Geometry check sheet. Reference: drawing and pictorial views, mm from the part's lowest x, y, z. A direction names the side the tool comes from. Give positions to 0.01 mm unless a question says otherwise; leave off trailing zeros. Order: outer loops, then holes, each group sorted by start corner. A loop starts at its lowest first (then second) coordinate and runs counter-clockwise, first axis right, second up. Notation, with made-up numbers: (67.5, -38.5) -> (97.5, -38.5) arc R33 ccw to (97.5, -0.5) -> close; hole circle Ø4 at (43, -36). An arc over 180 degrees is marked (long way). Write each question's results on one line, items separated by ' | '.
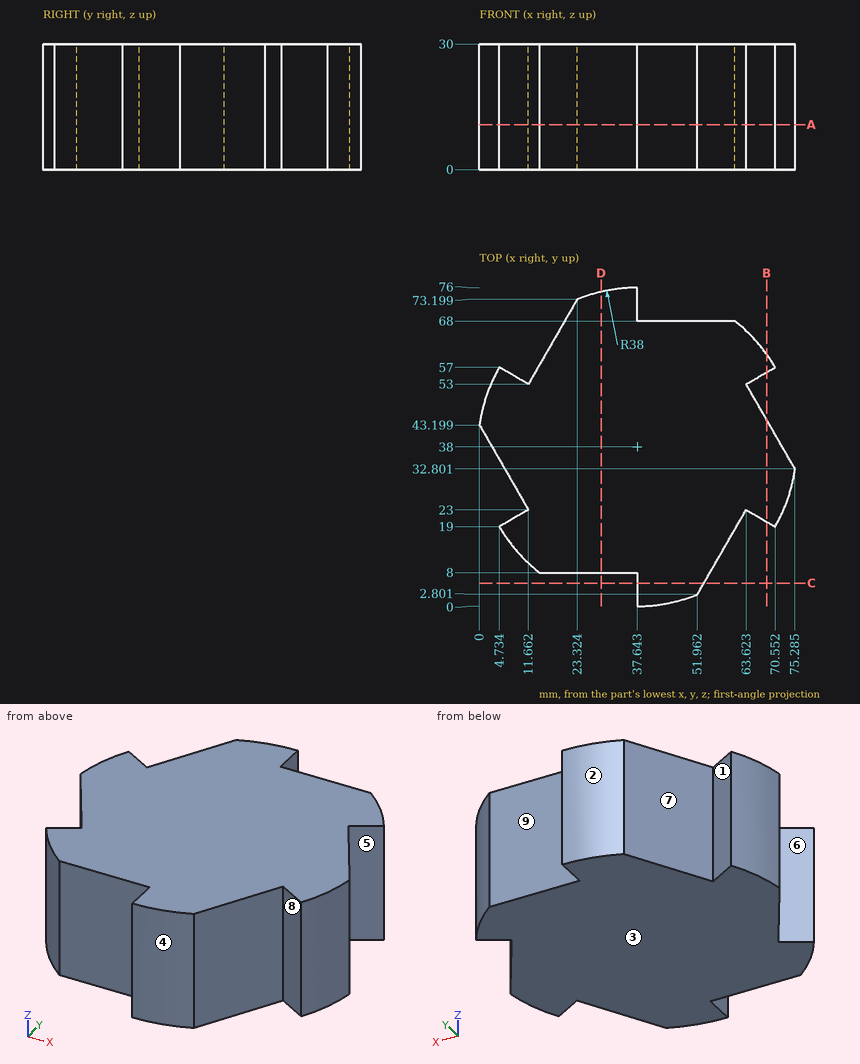
1. Mould release check, pull along X, two halves, no side actions. Record for the marked faces 1, 2, 3 and 4: +X half, -X half, draft (parallel to the pull), parting line (faces both ways), or undercut.
Verdict:
face 1: undercut | face 2: -X half | face 3: draft | face 4: +X half
2. Section check A-A on z = 10.75. Record the cut outline in (x, y) (1 decimal).
Verdict:
outline: (0, 43.2) -> (11.7, 23) -> (4.7, 19) arc R38 ccw to (14.3, 8) -> (37.6, 8) -> (37.6, 0) arc R38 ccw to (52, 2.8) -> (63.6, 23) -> (70.6, 19) arc R38 ccw to (75.3, 32.8) -> (63.6, 53) -> (70.6, 57) arc R38 ccw to (61, 68) -> (37.6, 68) -> (37.6, 76) arc R38 ccw to (23.3, 73.2) -> (11.7, 53) -> (4.7, 57) arc R38 ccw to start
3. Section check C-C on y = 5.5. Record the cut outline in (x, z).
Verdict:
outline: (37.64, 0) -> (53.52, 0) -> (53.52, 30) -> (37.64, 30) -> close
4. Gauge pin test, flat ends, axial feed: pin 1 Ø4 at (y, z) = (53.5, 16.5) entering from +X (1 decimal); pin 2 Ø2.5 at (y, z) = (72, 9) entering from +X; pin 3 Ø8 at (x, z) = (57.5, 7.5) entering from +Y. Record the tip position at first contact, or that the pin passes through.
Verdict:
pin 1: stops at x = 68 | pin 2: stops at x = 37.64 | pin 3: stops at y = 68
5. Material ranges on probe 1 along X at (y, z) = (21, 14.5) (1 decimal); probe 2 along Y at (x, z) = (70, 26.5) (1 decimal); probe 3 along Y at (x, z) = (8, 19) (1 decimal), recorded low to high. Write a range as from..to.
Verdict:
probe 1: x = 8.2..62.5, 67.1..71.6 | probe 2: y = 19.3..42, 56.7..57.9 | probe 3: y = 14.2..20.9, 29.3..55.1
6. Section check B-B on x = 68.5. Record the cut outline in (y, z) (1 decimal).
Verdict:
outline: (20.2, 0) -> (44.6, 0) -> (44.6, 30) -> (20.2, 30) -> close; (55.8, 0) -> (60.2, 0) -> (60.2, 30) -> (55.8, 30) -> close
7. Section check D-D on x = 29. Record the cut outline in (y, z) (1 decimal).
Verdict:
outline: (8, 0) -> (75, 0) -> (75, 30) -> (8, 30) -> close
8. Access from +Z, -Z, +X, -X, +Y, -Y to the whole of each face (thin tool, end or side, straight path). Record for the marked faces 5, 6, 7, 8 and 9.
Verdict:
face 5: +Z, -Z, +X | face 6: +Z, -Z, -X | face 7: +Z, -Z, +Y | face 8: +Z, -Z, -Y | face 9: +Z, -Z, +X, +Y
